from build123d import *

# Parameters (mm, degrees)
SKETCH1_R           = 57.15
BOSS_EXTRUDE1_DEPTH = 12.7
CUT_EXTRUDE1_START  = -11.1125
SKETCH2_R           = 57.15
SKETCH2_R_2         = 55.5625
CUT_EXTRUDE1_DEPTH  = 11.1125
SKETCH3_R           = 50.8
CUT_EXTRUDE2_DEPTH  = 9.525
SKETCH4_R           = 12.7
BOSS_EXTRUDE2_DEPTH = 6.35
CUT_EXTRUDE4_DEPTH  = 12.7
CHAMFER1_SIZE       = 0.79375


with BuildPart() as part:
    # Sketch1 → Boss-Extrude1 (new body)
    with BuildSketch(Plane.XY):
        Circle(SKETCH1_R)
    extrude(amount=BOSS_EXTRUDE1_DEPTH)

    # Sketch2 → Cut-Extrude1 (cut)
    with BuildSketch(Plane.XY.offset(12.7).offset(CUT_EXTRUDE1_START)):
        Circle(SKETCH2_R)
        Circle(SKETCH2_R_2, mode=Mode.SUBTRACT)
    extrude(amount=CUT_EXTRUDE1_DEPTH, mode=Mode.SUBTRACT)

    # Sketch3 → Cut-Extrude2 (cut)
    with BuildSketch(Plane(origin=(0, 0, 0), x_dir=(-1, 0, 0), z_dir=(0, 0, -1))):
        Circle(SKETCH3_R)
    extrude(amount=-CUT_EXTRUDE2_DEPTH, mode=Mode.SUBTRACT)

    # Sketch4 → Boss-Extrude2 (add)
    with BuildSketch(Plane(origin=(0, 0, 9.525), x_dir=(-1, 0, 0), z_dir=(0, 0, -1))):
        Circle(SKETCH4_R)
    extrude(amount=BOSS_EXTRUDE2_DEPTH)

    # Sketch6 → Cut-Extrude4 (cut)
    with BuildSketch(Plane(origin=(0, 0, 3.175), x_dir=(-1, 0, 0), z_dir=(0, 0, -1))):
        Polygon((7.332348419, 0), (3.666174209, 6.35), (-3.666174209, 6.35), (-7.332348419, 0), (-3.666174209, -6.35), (3.666174209, -6.35), align=None)
    extrude(amount=-CUT_EXTRUDE4_DEPTH, mode=Mode.SUBTRACT)

    # Chamfer1
    chamfer1_edges = [part.edges().sort_by_distance(p)[0] for p in [
        (12.7, 0, 3.175),
    ]]
    chamfer(chamfer1_edges, length=CHAMFER1_SIZE)


solid = part.part
Can you work these out from the model? Positions are in its coordinate system, mm. A direction names the side the tool comes from. Coordinates: 2 decimals unless noted, no trailing zeros. Loops run counter-clockwise (first coordinate to the right, second up) from the corner with the lowest first, then second, coordinate; pieces in that order, holes last. Notation, with made-up numbers: (2.25, 69.25) - (57.25, 69.25) arc R23 cw to (57.25, 78.25) - close; hole circle Ø9 at (74, 63). An arc over 180 degrees is marked (long way). Put each result on its own line as item: value. Start each with the question number.
Item 1: Suppose I cut it at D-D (x = -31). Please give me the cut outline in (y, z) (1 decimal).
Item 2: For pin 1 (6 mm diameter, centred on x = -0.5, z = 6, fed in from -Y); pin 2 (6 mm diameter, centred on x = 44.5, z = 11, fed in from -Y); pin 3 (6 mm diameter, centred on x = -1, z = 7.5, fed in from +Y), each with a flat end and sliding along its axis, tell me the tip position at first contact or that it passes through.
Item 3: If we mould it in two halves opening along Y, with no side actions, what happens to faces 4 (the face through (-7.23, 55.09, 7.07)), 5 (the face through (0, -6.35, 8)), 6 (the face through (-47, 30, 1.587))? For each: +Y half, -Y half, draft (parallel to the pull), parting line (faces both ways), or undercut.
Item 4: Suppose I cut it at C-C (y = 38.5). Please give me the cut outline in (x, z) (1 decimal), and give its area (3 significant figures).
Item 5: Suppose I cut it at A-A (z = 7.5). State how many separate pieces and enclosed holes the cut face has, and give its area (3 significant figures).
Item 6: If I drill on line 1 along Y through (x, z) = (0, 5); line 2 along Y through (x, z) = (0, 3.25); line 3 along Z through (x, y) = (-38.5, -1) (3 decimals), over which ranges is the centre line in solid material (lowest first)?
Item 7: Which directions (+Z, -Z, +X, -X, +Y, -Y) give clear straight access to the entire face, cutting with the end or side of a thin tool? Please do faces 1 (the face through (-1, -12, 12.7)), 2 (the face through (-5, -5, 3.175)), 3 (the face through (-5.474, -3.219, 7.871)).
Here are the results:
1. outline: (-48, 0) - (-40.2, 0) - (-40.2, 9.5) - (40.2, 9.5) - (40.2, 0) - (48, 0) - (48, 1.6) - (46.1, 1.6) - (46.1, 12.7) - (-46.1, 12.7) - (-46.1, 1.6) - (-48, 1.6) - close
2. pin 1: y = -55.56
2. pin 2: y = -36.95
2. pin 3: y = 55.56
3. face 4: parting line
3. face 5: undercut
3. face 6: draft
4. outline: (-42.2, 0) - (-33.1, 0) - (-33.1, 9.5) - (33.1, 9.5) - (33.1, 0) - (42.2, 0) - (42.2, 1.6) - (40.1, 1.6) - (40.1, 12.7) - (-40.1, 12.7) - (-40.1, 1.6) - (-42.2, 1.6) - close
4. area: 393 mm²
5. separate pieces: 2
5. enclosed holes: 2
5. area: 1,960 mm²
6. line 1: -55.56 to -50.8, -12.7 to -6.35, 6.35 to 12.7, 50.8 to 55.56
6. line 2: -55.56 to -50.8, -11.98 to -6.35, 6.35 to 11.98, 50.8 to 55.56
6. line 3: 9.525 to 12.7
7. face 1: +Z, +X, -X, +Y, -Y
7. face 2: -Z
7. face 3: +Z, -Z
